Could you check a few things on this model? Use its own coordinates, in mm. Face numbers are marked on the shaded views. A direction names the side the tool comes from. Round coordinates to 2 decimals unless told otherwise and drop trailing zeros. Loops run counter-clockwise (first coordinate to the right, second up) from the corner with the lowest first, then second, coordinate; pieces in that order, holes last. Notation, with made-up numbers: (-7.5, -28) -> (3.5, -28) arc R24 ccw to (3.5, -10) -> close; hole circle Ø3 at (19, 11). An arc over 180 degrees is marked (long way). One line per item, written item: value.
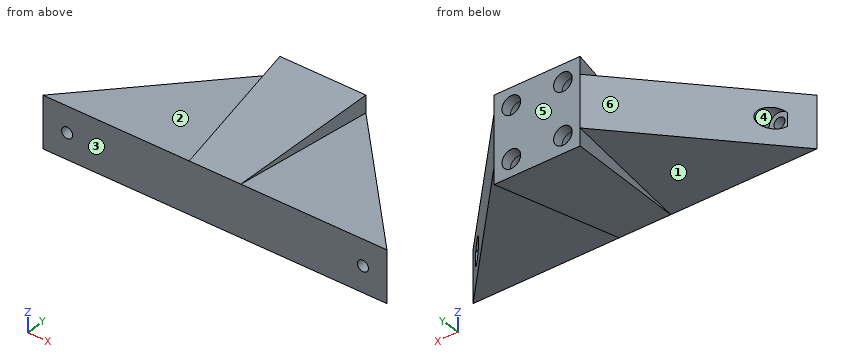
```python
from build123d import *

# Parameters (mm, degrees)
SKETCH2_W            = 15
SKETCH2_H            = 15
BOSS_EXTRUDE1_DEPTH  = 40
BOSS_EXTRUDE1_TAPER  = -7.125
SKETCH2_4_W          = 42.5
SKETCH2_4_H          = 15
BOSS_EXTRUDE4_DEPTH  = 40
CUT_EXTRUDE1_DEPTH   = 15
CUT_EXTRUDE2_START   = -5
SKETCH5_R            = 1.6
SKETCH5_R_2          = 3
CUT_EXTRUDE2_DEPTH   = 35
SKETCH5_3_R          = 1.6
CUT_EXTRUDE3_DEPTH   = 41.0000001
LPATTERN1_COUNT      = 2
LPATTERN1_PITCH      = 15
LPATTERN1_COUNT_DIR2 = 2
LPATTERN1_PITCH_DIR2 = 15


with BuildPart() as part:
    # Sketch2 → Boss-Extrude1 (new body)
    with BuildSketch(Plane(origin=(0, 0, 0), x_dir=(1, 0, 0), z_dir=(0, 1, 0))):
        Rectangle(SKETCH2_W, SKETCH2_H)
    extrude(amount=BOSS_EXTRUDE1_DEPTH, taper=BOSS_EXTRUDE1_TAPER)

    # Sketch2<4> → Boss-Extrude4 (add)
    with BuildSketch(Plane(origin=(0, 0, 0), x_dir=(1, 0, 0), z_dir=(0, 1, 0))):
        with Locations((-28.75, 0)):
            Rectangle(SKETCH2_4_W, SKETCH2_4_H)
        with Locations((28.75, 0)):
            Rectangle(SKETCH2_4_W, SKETCH2_4_H)
    extrude(amount=BOSS_EXTRUDE4_DEPTH)

    # Sketch4 → Cut-Extrude1 (cut)
    with BuildSketch(Plane(origin=(0, 0, -7.5), x_dir=(-1, 0, 0), z_dir=(0, 0, -1))):
        Polygon((-12.499988408, 40), (-50, 0), (-50, 40), align=None)
    cut_extrude1 = extrude(amount=-CUT_EXTRUDE1_DEPTH, mode=Mode.SUBTRACT)

    # Sketch5 → Cut-Extrude2 (cut)
    with BuildSketch(Plane.XZ.offset(CUT_EXTRUDE2_START)):
        with Locations((43, 0)):
            Circle(SKETCH5_R)
        with Locations((43, 0)):
            Circle(SKETCH5_R_2)
        with Locations((43, 0)):
            Circle(SKETCH5_R, mode=Mode.SUBTRACT)
    cut_extrude2 = extrude(amount=-CUT_EXTRUDE2_DEPTH, mode=Mode.SUBTRACT)

    # Sketch5<3> → Cut-Extrude3 (cut, through all)
    with BuildSketch(Plane.XZ):
        with Locations((43, 0)):
            Circle(SKETCH5_3_R)
    cut_extrude3 = extrude(amount=-CUT_EXTRUDE3_DEPTH, mode=Mode.SUBTRACT)

    # Mirror1: Cut-Extrude1, Cut-Extrude2, Cut-Extrude3 across plane
    add(cut_extrude1.mirror(Plane(origin=(0, 0, 0), x_dir=(0, 0, 1), z_dir=(1, 0, 0))), mode=Mode.SUBTRACT)
    add(cut_extrude2.mirror(Plane(origin=(0, 0, 0), x_dir=(0, 0, 1), z_dir=(1, 0, 0))), mode=Mode.SUBTRACT)
    add(cut_extrude3.mirror(Plane(origin=(0, 0, 0), x_dir=(0, 0, 1), z_dir=(1, 0, 0))), mode=Mode.SUBTRACT)

    # Sketch8 → CSK for M3 Oval Head Machine Screw1 (revolve, cut)
    with BuildSketch(Plane(origin=(-7.499988408, 40, -7.499988408), x_dir=(0, 0, 1), z_dir=(1, 0, 0))):
        Polygon((0, 0), (0, 11.502151548), (2.5, 10), (2.5, 2.860133251), (2.7, 0), align=None)
    csk_for_m3_oval_head_machine_screw1 = revolve(axis=Axis((-7.499988408, 46.35, -7.499988408), (0, -1, 0)), mode=Mode.SUBTRACT)

    # LPattern1: CSK for M3 Oval Head Machine Screw1 2 × 2
    with Locations(*[(j * LPATTERN1_PITCH_DIR2, 0, i * LPATTERN1_PITCH) for i in range(LPATTERN1_COUNT) for j in range(LPATTERN1_COUNT_DIR2) if (i, j) != (0, 0)]):
        add(csk_for_m3_oval_head_machine_screw1, mode=Mode.SUBTRACT)


solid = part.part
```
(1) Imagine slicing it at C-C on x = 31. Write out the boundary of the cut face in (y, z).
Results below:
outline: (0, -7.5) -> (20.27, -7.5) -> (20.27, 7.5) -> (0, 7.5) -> close
(2) We'd pull the mould along X, two halves only. Please class the marked faces 4, 5 and 6: +X half, -X half, draft (parallel to the pull), parting line (faces both ways), or undercut.
Results below:
face 4: undercut
face 5: draft
face 6: -X half
(3) Please list where these lines run through material, in increasing order: L1, parallel to X at y = 36.5, z = -5.5; L2, parallel to X at y = 33.5, z = -6.25; L3, parallel to Z at x = 21.5, y = 8.5.
Results below:
L1: x = -15.78 to -9, -6 to 6, 9 to 15.78
L2: x = -18.59 to -9.67, -5.33 to 5.33, 9.67 to 18.59
L3: z = -7.5 to 7.5
(4) Imagine slicing it at A-A on x = -43. Write out the boundary of the cut face in (y, z).
Results below:
outline: (0, -7.5) -> (7.47, -7.5) -> (7.47, -3) -> (5, -3) -> (5, -1.6) -> (0, -1.6) -> close; (0, 1.6) -> (5, 1.6) -> (5, 3) -> (7.47, 3) -> (7.47, 7.5) -> (0, 7.5) -> close
(5) For pin 1 Ø4 at (x, y) = (10, 23.5) entering from -Z; pin 2 Ø5 at (x, z) = (36, -1.5) entering from +Y; pin 3 Ø20 at (x, y) = (34, 16) entering from -Z, each with a flat end and sliding along its axis, tell me the tip position at first contact or that it passes through.
Results below:
pin 1: stops at z = -10.69
pin 2: stops at y = 17.6
pin 3: stops at z = -7.5
(6) On a 3-axis mill with a long thin cutter (end or side, diameter ignored), from which of +Z, -Z, +X, -X, +Y, -Y can I reach the whole of each face in a straight line? I mean the marked faces 1, 2 and 3. Say none if no direction works.
Results below:
face 1: -Z, -X, -Y
face 2: +Z, -X, -Y
face 3: +Z, -Z, +X, -X, -Y
(7) Imagine slicing it at B-B on y = 33. Give the number of separate pieces and of enclosed holes in the cut face, then the cut area to 3 significant figures.
Results below:
separate pieces: 1
enclosed holes: 4
area: 685 mm²
